Part model, mm, in its own coordinate system. Round coordinates to 2 decimals unless told otherwise and drop trailing zeros. Write each loop counter-clockwise with the first axis right and the second up, starting at its lowest first coordinate (ties: lowest second). Pieces come first, ordered by that corner, then holes. Notation, with made-up numbers: M -28,-39.5 L 23,-39.5 A11 cw 23,-25.5 Z; hole C 60,-19.75 d6. An arc over 180 degrees is marked long. Use a Markdown table: item, result. Add a question column.
1) Slice it at C-C on x = 2.5. Write the cut outline in (y, z).
2) Drop flat-ended pins along their axis: P1, Ø5.5, axis at x = 63.5, y = 0, coming from the -Z side; P2, Ø3, axis at y = 3.5, z = 2.5, coming from the -X side. Give the stop position or say it passes through.
3) Slice it at B-B on z = 2.75. Give the number of separate pieces and of enclosed holes in the cut face, plus the area to 3 significant figures.
4) Wall check: probe 1 along X at (y, z) = (1, 3.75); probe 2 along X at (y, z) = (1.5, 3.25); probe 3 along Y at (x, z) = (-63.5, 2.5). Give the ranges that are in metal, low to high.
5) Slice it at A-A on y = 0. Write the cut outline in (x, z), plus the area to 3 significant figures.
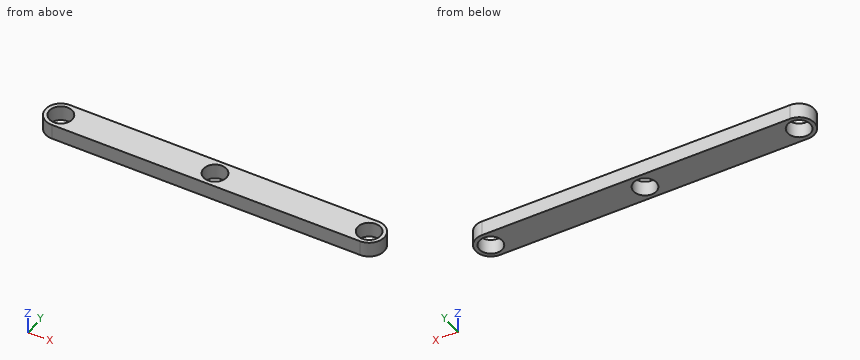
```python
from build123d import *

# Parameters (mm, degrees)
BOSS_EXTRUDE1_DEPTH            = 6.35
F_4_0_375_DIAMETER_HOLE1_D     = 9.525
F_4_0_375_DIAMETER_HOLE1_DEPTH = 6.35


with BuildPart() as part:
    # Sketch1 → Boss-Extrude1 (new body)
    with BuildSketch(Plane.XY):
        with BuildLine():
            Line((-63.5, -6.35), (63.5, -6.35))
            ThreePointArc((63.5, -6.35), (69.85, 0), (63.5, 6.35))
            Line((63.5, 6.35), (-63.5, 6.35))
            ThreePointArc((-63.5, 6.35), (-69.85, 0), (-63.5, -6.35))
        make_face()
    extrude(amount=BOSS_EXTRUDE1_DEPTH)

    # #4 (0.375) Diameter Hole1
    with Locations(Plane.XY.offset(6.35)):
        with Locations((0, 0), (-63.5, 0), (63.5, 0)):
            Hole(F_4_0_375_DIAMETER_HOLE1_D / 2, depth=F_4_0_375_DIAMETER_HOLE1_DEPTH)


solid = part.part
```
Entries:
| question | item | result |
|---|---|---|
| 1 | outline | M -6.35,0 L -4.05,0 L -4.05,6.35 L -6.35,6.35 Z; M 4.05,0 L 6.35,0 L 6.35,6.35 L 4.05,6.35 Z |
| 2 | P1 | passes through |
| 2 | P2 | stops at x = -69.53 |
| 3 | separate pieces | 1 |
| 3 | enclosed holes | 3 |
| 3 | area | 1,530 mm^2 |
| 4 | probe 1 | x = -69.77 to -68.16, -58.84 to -4.66, 4.66 to 58.84, 68.16 to 69.77 |
| 4 | probe 2 | x = -69.67 to -68.02, -58.98 to -4.52, 4.52 to 58.98, 68.02 to 69.67 |
| 4 | probe 3 | y = -6.35 to -4.76, 4.76 to 6.35 |
| 5 | outline | M -69.85,0 L -68.26,0 L -68.26,6.35 L -69.85,6.35 Z; M -58.74,0 L -4.76,0 L -4.76,6.35 L -58.74,6.35 Z; M 4.76,0 L 58.74,0 L 58.74,6.35 L 4.76,6.35 Z; M 68.26,0 L 69.85,0 L 69.85,6.35 L 68.26,6.35 Z |
| 5 | area | 706 mm^2 |
